Autodesk Inventor part; units mm, degrees
ref_plane "YZ Plane" through (0, 0, 0) normal (1, 0, 0) x (0, 1, 0)
ref_plane "XZ Plane" through (0, 0, 0) normal (0, 1, 0) x (-1, 0, 0)
ref_plane "XY Plane" through (0, 0, 0) normal (0, 0, 1) x (1, 0, 0)
sketch "Skizze1" plane through (0, 0, 0) normal (0, 0, 1) x (1, 0, 0)
  circle A0 centre (5.8119, 6.7241) radius 1.5
  circle A1 centre (7.8119, 6.7241) radius 5.5
  line L0 (2.3119, 6.7241) -> (2.3119, 24.7241)
  line L1 (4.3119, 26.7241) -> (5.3119, 26.7241)
  line L2 (5.3119, 26.7241) -> (12.8762, 8.8696)
  arc A2 (4.3119, 26.7241) -> (2.3119, 24.7241) centre (4.3119, 24.7241) ccw
  circle A3 centre (5.8119, 6.7241) radius 1.7
  point P0 (0, 0)
  point P1 (2.3119, 26.7241)
  dimension "d0" = 20
  dimension "d1" = 3
  dimension "d2" = 2
  dimension "d3" = 2
  dimension "d6" = 0.2
  dimension "d14" = 11
extrude "Extrusion1" add sketch "Skizze1" along normal blind 22 contours A1 | A1 L0 A2 L1 L2
fillet "Rundung1" radius 2 1 edges at (5.3119, 26.7241, 11)
sketch "Skizze2" plane through (0, 0, 0) normal (0, 0, -1) x (-1, 0, 0)
  circle A0 centre (-5.8119, 6.7241) radius 1.7
  arc A1 (-2.3119, 23.9575) -> (-6.1535, 24.7377) centre (-4.3119, 23.9575) ccw
  line L0 (-12.8762, 8.8696) -> (-6.1535, 24.7377)
  arc A2 (-12.8762, 8.8696) -> (-2.3119, 6.7241) centre (-7.8119, 6.7241) ccw
  line L1 (-2.3119, 23.9575) -> (-2.3119, 6.7241)
  circle A3 centre (-4.5041, 21.3778) radius 1.45
  point P0 (0, 0)
  dimension "d8" = 2.9
extrude "Extrusion2" cut sketch "Skizze2" against normal blind 4 contours A3
sketch "Skizze3" plane through (0, 0, 22) normal (0, 0, 1) x (1, 0, 0)
  circle A0 centre (4.5041, 21.3778) radius 1.45
  point P0 (0, 0)
extrude "Extrusion3" cut sketch "Skizze3" against normal blind 4
ref_plane "Arbeitsebene1" through (50, 0, 23) normal (0, 0, -1) x (-1, 0, 0)
sketch "Skizze4" plane through (50, 0, 23) normal (0, 0, -1) x (-1, 0, 0)
  circle A0 centre (45.4959, 21.3778) radius 1.45
  circle A1 centre (44.1881, 6.7241) radius 1.7
  circle A2 centre (44.1881, 6.7241) radius 1.7
  circle A3 centre (45.4959, 21.3778) radius 1.45
  circle A4 centre (44.1881, 6.7241) radius 14.712
  circle A5 centre (29.4761, 6.7241) radius 1.45
  point P0 (50, 0)
  dimension "d13" = 2.9
sketch "Skizze5" plane through (12.8762, 8.8696, 22) normal (0.9208, 0.3901, 0) x (0, 0, -1)
  line L0 (0, 17.2334) -> (22, 17.2334)
  line L1 (0, 0) -> (0, 17.2334)
  line L2 (22, 0) -> (0, 0)
  line L3 (22, 0) -> (22, 17.2334)
  circle A0 centre (11, 14.4172) radius 1.4
  point P0 (22, -3.1439)
  dimension "d15" = 2.8
extrude "Extrusion4" cut sketch "Skizze5" against normal blind 10 contours A0
properties part number "Anglerfish_coverslipclamp_levelarm"
Geometry: final body of the model. Coordinates: model frame, mm. A direction names the side the tool comes from. Give positions to 0.01 mm unless a question says otherwise; leave off trailing zeros. Order: outer loops, then holes, each group sorted by start corner. A loop starts at its lowest first (then second) coordinate and runs counter-clockwise, first axis right, second up. Notation, with made-up numbers: M -27,-37 L 20,-37 A12 cw 20,-30 Z; hole C 45,36 d10. An arc over 180 degrees is marked long. Answer as CSV lines item,"result". Start each with the question number.
1) Mould query, pull axis Z, two halves, no side actions, for faces 4 (the cylindrical face through (5.08, 19.74, 11.3)), 5 (the cylindrical face through (9.04, 1.363, 10.846)), 6 (the flat face through (7, 11, 22)). Classes: +Z half, -Z half, draft (parallel to the pull), parting line (faces both ways), or undercut.
2) First-contact query: P1, Ø1.5, axis at y = 4, z = 5.5, coming from the -X side; P2, Ø8, axis at y = 16, z = 5.5, coming from the +X side; P3, Ø4, axis at y = 4.5, z = 17.5, coming from the -X side. Flat tips, straight axial feed; report the tip coordinate or a pass-through.
3) Cut plane A-A (z = 10.75). State how many separate pieces and enclosed holes the cut face has, then the cut area to 3 significant figures.
4) Cut plane B-B (x = 11.5). Output: boundary loops of the cut face in (y, z), then the cut area to 3 significant figures.
5) Line query: line 1 (Y direction, x = 5.25, z = 12.25); line 2 (Y direction, x = 5, z = 10.75); line 3 (Y direction, x = 3.25, z = 19.75). Output: solid intervals per line, ascending. Write a range as from..to.
6) Set-up query: faces 1 (the cylindrical face through (3.44, 22.36, 20.03)), 2 (the cylindrical face through (7.433, 6.213, 10.846)), 3 (the flat face through (5, 21, 4)). Return all of +Z, -Z, +X, -X, +Y, -Y with unobstructed straight access to the full face (end or side cutting, diameter ignored); none if empty.
7) Cut plane C-C (y = 17.5). Output: boundary loops of the cut face in (x, z), then the cut area to 3 significant figures.
Findings below:
1,face 4,"undercut"
1,face 5,"draft"
1,face 6,"+Z half"
2,P1,"stops at x = 2.68"
2,P2,"stops at x = 11.55"
2,P3,"stops at x = 2.32"
3,separate pieces,"2"
3,enclosed holes,"1"
3,area,"164 mm²"
4,outline,"M 2.64,0 L 12.12,0 L 12.12,22 L 2.64,22 Z"
4,area,"208 mm²"
5,line 1,"y = 1.86..5.12, 8.33..20.61, 21.98..25.73"
5,line 2,"y = 2..5.23, 8.22..19.69, 22.69..25.84"
5,line 3,"y = 3.65..20.65, 22.11..25.65"
6,face 1,"+Z"
6,face 2,"+Z, -Z"
6,face 3,"-Z"
7,outline,"M 2.31,0 L 9.22,0 L 9.22,22 L 2.31,22 Z"
7,area,"152 mm²"
